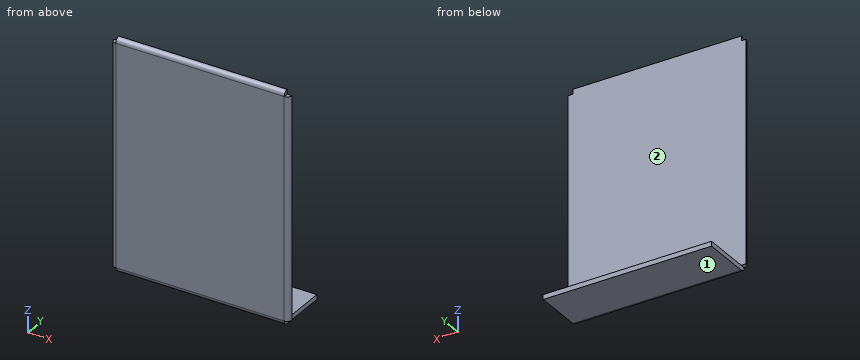
```python
from build123d import *

# Parameters (mm, degrees)
BOTTOM_SIDE_W       = 71
BOTTOM_SIDE_H       = 93
BOTTOM_EXTR_DEPTH   = 2
X_CORNER_W          = 93
X_CORNER_H          = 2
X_CORNER_REV_ANGLE  = 90
Z_CORNER_W          = 71
Z_CORNER_H          = 2
Z_CORNER_REV_ANGLE  = 90
X0_CORNER_W         = 93
X0_CORNER_H         = 2
X0_CORNER_REV_ANGLE = 90
Z0_CORNER_W         = 71
Z0_CORNER_H         = 2
Z0_CORNER_REV_ANGLE = 90
Z0_SIDE_W           = 71
Z0_SIDE_H           = 2
Z0_EXTR_DEPTH       = 20


with BuildPart() as part:
    # bottom side → bottom extr (new body)
    with BuildSketch(Plane(origin=(0, 0, 0), x_dir=(1, 0, 0), z_dir=(0, 1, 0))):
        with Locations((35.5, 46.5)):
            Rectangle(BOTTOM_SIDE_W, BOTTOM_SIDE_H)
    extrude(amount=BOTTOM_EXTR_DEPTH)

    # X+ corner → X+ corner rev (revolve)
    with BuildSketch(Plane(origin=(71, 0, 0), x_dir=(0, 0, -1), z_dir=(1, 0, 0))):
        with Locations((46.5, 1)):
            Rectangle(X_CORNER_W, X_CORNER_H)
    revolve(axis=Axis((71, 2, 0), (0, 0, 1)), revolution_arc=X_CORNER_REV_ANGLE)

    # Z+ corner → Z+ corner rev (revolve)
    with BuildSketch(Plane.XY):
        with Locations((35.5, 1)):
            Rectangle(Z_CORNER_W, Z_CORNER_H)
    revolve(axis=Axis((0, 2, 0), (-1, 0, 0)), revolution_arc=Z_CORNER_REV_ANGLE)

    # X0 corner → X0 corner rev (revolve)
    with BuildSketch(Plane.ZY):
        with Locations((-46.5, 1)):
            Rectangle(X0_CORNER_W, X0_CORNER_H)
    revolve(axis=Axis((0, 2, -93), (0, 0, -1)), revolution_arc=X0_CORNER_REV_ANGLE)

    # Z0 corner → Z0 corner rev (revolve)
    with BuildSketch(Plane(origin=(0, 0, -93), x_dir=(-1, 0, 0), z_dir=(0, 0, -1))):
        with Locations((-35.5, 1)):
            Rectangle(Z0_CORNER_W, Z0_CORNER_H)
    revolve(axis=Axis((71, 2, -93), (1, 0, 0)), revolution_arc=Z0_CORNER_REV_ANGLE)

    # Z0 side → Z0 extr (add)
    with BuildSketch(Plane(origin=(0, 2, 0), x_dir=(1, 0, 0), z_dir=(0, 1, 0))):
        with Locations((35.5, 94)):
            Rectangle(Z0_SIDE_W, Z0_SIDE_H)
    extrude(amount=Z0_EXTR_DEPTH)


solid = part.part
```
Here's how the part is built. I have some questions about the finished solid (model axes, mm). Face numbers are marked on the shaded views. A direction names the side the tool comes from. Coordinates: 2 decimals unless noted, no trailing zeros. Write each loop counter-clockwise with the first axis right and the second up, starting at its lowest first coordinate (ties: lowest second). Pieces come first, ordered by that corner, then holes. Notation, with made-up numbers: (2.25, 56) -> (26.25, 56) arc R23 cw to (26.25, 82) -> close; hole circle Ø8 at (84.5, -17.75). An arc over 180 degrees is marked (long way). Use a Markdown table: item, result. Add a question column.
(1) If we section it at C-C, the plane z = -17: Write out the boundary of the cut face in (x, y).
(2) For the marked faces 1 and 2, which set-ups out of +Z, -Z, +X, -X, +Y, -Y let a thin tool reach every point of the face, with its end or its side?
(3) Please list where these lines run through material, in increasing order: line 1 (Y direction, x = 70.5, z = -89.5); line 2 (Z direction, x = 9, y = 12); line 3 (X direction, y = 1.75, z = -85).
(4) If we section it at A-A, the plane x = 14.5: Write out the boundary of the cut face in (y, z).
(5) If we section it at B-B, the plane y = 14: Write out the boundary of the cut face in (x, z), and give its area (3 significant figures).
(6) I'm going to push flat-ended pins straight in: P1, Ø10, axis at x = 38, y = 15, coming from the +Z side; P2, Ø2, axis at x = 72.5, y = 1.5, coming from the -Z side; P3, Ø1, axis at y = 1, z = 1, coming from the -X side. Where does each tip first touch, or does it pass through?
Outcome:
| question | item | result |
|---|---|---|
| 1 | outline | (-2, 2) arc R2 ccw to (0, 0) -> (71, 0) arc R2 ccw to (73, 2) -> close |
| 2 | face 1 | -Z, +X, -X, +Y, -Y |
| 2 | face 2 | +Z, +X, -X, +Y |
| 3 | line 1 | y = 0 to 2 |
| 3 | line 2 | z = -95 to -93 |
| 3 | line 3 | x = -1.98 to 72.98 |
| 4 | outline | (0, -93) arc R2 ccw to (2, -95) -> (22, -95) -> (22, -93) -> (2, -93) -> (2, 2) arc R2 ccw to (0, 0) -> close |
| 5 | outline | (0, -95) -> (71, -95) -> (71, -93) -> (0, -93) -> close |
| 5 | area | 142 mm^2 |
| 6 | P1 | stops at z = -93 |
| 6 | P2 | stops at z = -93 |
| 6 | P3 | stops at x = 0 |
